Part model, mm, in its own coordinate system. Round coordinates to 2 decimals unless told otherwise and drop trailing zeros. Loops run counter-clockwise (first coordinate to the right, second up) from the corner with the lowest first, then second, coordinate; pieces in that order, holes last. Notation, with made-up numbers: (14.25, -33) - (65.25, -33) arc R16 ccw to (65.25, -19) - close; hole circle Ø1 at (-3.5, 87). An arc over 180 degrees is marked (long way). Put each result on its own line as item: value.
Autodesk Inventor part; units mm, degrees
ref_plane "YZ Plane" through (0, 0, 0) normal (1, 0, 0) x (0, 1, 0)
ref_plane "XZ Plane" through (0, 0, 0) normal (0, 1, 0) x (-1, 0, 0)
ref_plane "XY Plane" through (0, 0, 0) normal (0, 0, 1) x (1, 0, 0)
sketch "Эскиз1" plane through (0, 0, 0) normal (0, 0, 1) x (1, 0, 0)
  circle A0 centre (0, 10.0167) radius 1.6
  line L0 (25.2327, 9.549) -> (31.7335, -1.7106)
  arc A1 (11.3933, 4.2802) -> (25.2327, 9.549) centre (0, 55.0167) ccw
  line L1 (11.3933, 4.2802) -> (2.8284, 12.8451)
  arc A2 (2.8284, 12.8451) -> (-2.8284, 12.8451) centre (0, 10.0167) ccw
  line L2 (-2.8284, 12.8451) -> (-11.3933, 4.2802)
  arc A3 (-25.2327, 9.549) -> (-11.3933, 4.2802) centre (0, 55.0167) ccw
  line L3 (-31.7335, -1.7106) -> (-25.2327, 9.549)
  arc A4 (-31.7335, -1.7106) -> (31.7335, -1.7106) centre (0, 55.0167) ccw
  arc A5 (1.9935, 28.8226) -> (-1.9935, 28.8226) centre (0, 28.6617) ccw
  line L4 (-1.9935, 28.8226) -> (-3.4887, 10.2982)
  arc A6 (-3.4887, 10.2982) -> (3.4887, 10.2982) centre (0, 10.0167) ccw
  line L5 (3.4887, 10.2982) -> (1.9935, 28.8226)
  circle A7 centre (0, 28.6617) radius 1.1
  circle A8 centre (0, 10.0167) radius 0.95
  circle A9 centre (0, 28.6617) radius 1.6
  circle A10 centre (0, 10.0167) radius 2.1
  circle A11 centre (0, 10.0167) radius 4
  circle A12 centre (0, 28.6617) radius 2.5
  line L6 (-2.4919, 28.8628) -> (-3.987, 10.3385)
  line L7 (3.987, 10.3385) -> (2.4919, 28.8628)
  point P0 (0, 0)
  dimension "d0" = 3.2
  dimension "d1" = 4.2
  dimension "d2" = 8
  dimension "d3" = 5
extrude "Выдавливание1" add sketch "Эскиз1" along normal blind 3.2 contours L7 A11 L5 L1 | L1 L5 A12 L7 | L5 A11 L1 | L1 A2 L2 L4 A12 L5 | A11 L4 A6 L5 | A12 L5 A5 L4 | A11 L5 A6 L4 A2 | A12 L4 A5 L5 | A12 L4 L2 L6 | L2 L4 A11 L6 | A11 L4 L2 | A9
sketch "Эскиз2" plane through (0, 0, 0) normal (0, 0, -1) x (-1, 0, 0)
  line L0 (0, 6.9767) -> (0, 71.9606)
  line L1 (-1.9935, 28.8226) -> (-3.4887, 10.2982)
  arc A0 (-3.4887, 10.2982) -> (3.4887, 10.2982) centre (0, 10.0167) ccw
  line L2 (3.4887, 10.2982) -> (1.9935, 28.8226)
  arc A1 (1.9935, 28.8226) -> (-1.9935, 28.8226) centre (0, 28.6617) ccw
  circle A2 centre (0, 10.0167) radius 1.925
  circle A3 centre (0, 28.6617) radius 1.1
  circle A4 centre (0, 28.6617) radius 1.1
  circle A5 centre (0, 10.0167) radius 2.1
  arc A6 (-3.987, 10.3385) -> (3.987, 10.3385) centre (0, 10.0167) ccw
  line L3 (2.4919, 28.8628) -> (3.987, 10.3385)
  arc A7 (2.4919, 28.8628) -> (-2.4919, 28.8628) centre (0, 28.6617) ccw
  line L4 (-3.987, 10.3385) -> (-2.4919, 28.8628)
  circle A8 centre (0, 28.6617) radius 2.5
  point P0 (0, 0)
  point P1 (-2.4919, 28.8628)
extrude "Выдавливание2" add sketch "Эскиз2" along normal blind 2.8 contours A8 L1 A1 L0 A3 | L0 A3 A1 L2 A8 | A8 A7 L0 A1 L1 | L2 A1 L0 A7 A8
properties part number "shatun"
1. Pin check, flat tips, straight feed: P1, Ø1, axis at x = -3, z = 2, coming from the -Y side; P2, Ø1, axis at y = 20, z = 2, coming from the -X side; P3, Ø1, axis at y = 28, z = 1.5, coming from the -X side. Stop position of each tip, or through.
A:
P1: stops at y = 6.89
P2: stops at x = -3.25
P3: stops at x = -2.6
2. Band-saw the part on D-D (z = -0.25). List the corners of the cut face in (x, y), plus the area to 3 significant figures.
A:
outline: circle Ø5 at (0, 28.66); hole circle Ø2.2 at (0, 28.66)
area: 15.8 mm²
3. Band-saw the part on C-C (z = 2.6). List the corners of the cut face in (x, y), plus the area to 3 significant figures.
A:
outline: (-3.99, 10.34) arc R4 ccw (long way) to (3.99, 10.34) - (2.49, 28.86) arc R2.5 ccw to (-2.49, 28.86) - close; hole circle Ø4.2 at (0, 10.02); hole circle Ø2.2 at (0, 28.66)
area: 139 mm²
4. Band-saw the part on B-B (y = 11.25). List the corners of the cut face in (x, z), plus the area to 3 significant figures.
A:
outline: (-3.91, 0) - (-1.7, 0) - (-1.7, 3.2) - (-3.91, 3.2) - close; (1.7, 0) - (3.91, 0) - (3.91, 3.2) - (1.7, 3.2) - close
area: 14.2 mm²
5. Band-saw the part on A-A (x = 0). List the corners of the cut face in (y, z).
A:
outline: (6.02, 0) - (7.92, 0) - (7.92, 3.2) - (6.02, 3.2) - close; (12.12, 0) - (26.16, 0) - (26.16, -2.8) - (27.56, -2.8) - (27.56, 3.2) - (12.12, 3.2) - close; (29.76, -2.8) - (31.16, -2.8) - (31.16, 3.2) - (29.76, 3.2) - close
6. Two-plate mould, pull along X, no slides. Class faces 1 (the cylindrical face through (-0.455, 12.067, 1.578)), 2 (the flat face through (0, 19, 3.2)), 3 (the flat face through (-3.23, 19.73, 1.58)): pulls with the +X half, pulls with the -X half, needs draft (parallel to the pull), parting line crosses it, or undercut.
A:
face 1: undercut
face 2: needs draft
face 3: pulls with the -X half
7. Probe line 1 along Y through (x, z) = (0.25, 1.2); line 2 along Y through (x, z) = (0, -1.35); line 3 along Z through (x, y) = (2.5, 28.25). List the from-to ranges inside material, lowest first. Write a range as [from, to].
A:
line 1: y = [6.02, 7.93], [12.1, 27.59], [29.73, 31.15]
line 2: y = [26.16, 27.56], [29.76, 31.16]
line 3: z = [0, 3.2]
